from build123d import *

# Parameters (mm, degrees)
MOUNT_SKETCH_W       = 18
MOUNT_SKETCH_H       = 7.25
PIN_HOLE_SKETCH_W    = 3
PIN_HOLE_SKETCH_H    = 9.25
PIN_HOLES_X2_COUNT   = 2
SCREW_HOLE_SKETCH_W  = 1.65
SCREW_HOLE_SKETCH_H  = 9.25
SCREW_HOLES_X8_COUNT = 8


with BuildPart() as part:
    # Mount Sketch → Mount (revolve)
    with BuildSketch(Plane.XY, mode=Mode.PRIVATE) as mount_sk:
        with Locations((-48, 95.625)):
            Rectangle(MOUNT_SKETCH_W, MOUNT_SKETCH_H)
    revolve(mount_sk.sketch.rotate(Axis((-108, 0, 0), (1, 0, 0)), 90), axis=Axis((-108, 0, 0), (1, 0, 0)))

    # Pin Hole Sketch → Pin Hole (revolve, cut)
    with BuildSketch(Plane.XY, mode=Mode.PRIVATE) as pin_hole_sk:
        with Locations((-46.5, 95.625)):
            Rectangle(PIN_HOLE_SKETCH_W, PIN_HOLE_SKETCH_H)
    pin_hole = revolve(pin_hole_sk.sketch.rotate(Axis((-48, 82, 0), (0, 1, 0)), 90), axis=Axis((-48, 82, 0), (0, 1, 0)), mode=Mode.SUBTRACT)

    # Pin Holes x2: Pin Hole ×2 about axis
    pin_holes_x2_axis = Axis((-38.1, 0, 0), (-1, 0, 0))
    for i in range(1, PIN_HOLES_X2_COUNT):
        add(pin_hole.rotate(pin_holes_x2_axis, i * 360 / PIN_HOLES_X2_COUNT), mode=Mode.SUBTRACT)

    # Screw Hole Sketch → Screw Hole (revolve, cut)
    with BuildSketch(Plane.XY, mode=Mode.PRIVATE) as screw_hole_sk:
        with Locations((-41.175, 95.625)):
            Rectangle(SCREW_HOLE_SKETCH_W, SCREW_HOLE_SKETCH_H)
    screw_hole = revolve(screw_hole_sk.sketch.rotate(Axis((-42, 82, 0), (0, 1, 0)), 90), axis=Axis((-42, 82, 0), (0, 1, 0)), mode=Mode.SUBTRACT)

    # Screw Holes x8: Screw Hole ×8 about axis
    screw_holes_x8_axis = Axis((-38.1, 0, 0), (-1, 0, 0))
    for i in range(1, SCREW_HOLES_X8_COUNT):
        add(screw_hole.rotate(screw_holes_x8_axis, i * 360 / SCREW_HOLES_X8_COUNT), mode=Mode.SUBTRACT)


solid = part.part
Here's how the part is built. I have some questions about the finished solid (model axes, mm). Coordinates: 2 decimals unless noted, no trailing zeros. Order: outer loops, then holes, each group sorted by start corner. A loop starts at its lowest first (then second) coordinate and runs counter-clockwise, first axis right, second up.
Item 1: If we section it at B-B on z = 19.5: List the corners of the cut face in (x, y) for me, plus the area to 3 significant figures.
Result sheet:
outline: (-57, -97.32) - (-39, -97.32) - (-39, -89.91) - (-57, -89.91) - close; (-57, 89.91) - (-39, 89.91) - (-39, 97.32) - (-57, 97.32) - close
area: 267 mm2
Item 2: For P1, Ø5, axis at x = -44, y = 44, coming from the -Z side; P2, Ø2, axis at x = -43.5, z = 60.5, coming from the +Y side; P3, Ø5, axis at x = -52.5, y = 15.5, coming from the +Z side; P4, Ø3.5, axis at x = -48, z = 0, coming from the +Y side, each with a flat end and sliding along its axis, tell me the tip position at first contact or that it passes through.
Result sheet:
P1: stops at z = -90.16
P2: stops at y = 79.44
P3: stops at z = 98.39
P4: passes through
Item 3: If we section it at A-A on y = 29: List the corners of the cut face in (x, z) for me, plus the area to 3 significant figures.
Result sheet:
outline: (-57, -94.92) - (-39, -94.92) - (-39, -87.31) - (-57, -87.31) - close; (-57, 87.31) - (-39, 87.31) - (-39, 94.92) - (-57, 94.92) - close
area: 274 mm2
Item 4: I need wall thicknesses on line 1 (X direction, y = 94, z = 0); line 2 (Y direction, x = -52.5, z = -40); line 3 (Z direction, x = -40, y = -64). Which ranges of each line are inside material? Lowest first, please.
Result sheet:
line 1: x = -57 to -51, -45 to -43.65, -40.35 to -39
line 2: y = -90.83 to -82.85, 82.85 to 90.83
line 3: z = -75.86 to -66.09, 66.09 to 75.86
Item 5: If we mould it in two halves opening along Y, with no side actions, what happens to faces 1 (the face through (-39, 29, -88)), 2 (the face through (-47.874, -29.812, 94.667)), 3 (the face through (-43.636, -67.8, 67.496))? For each: +Y half, -Y half, draft (parallel to the pull), parting line (faces both ways), or undercut.
Result sheet:
face 1: draft
face 2: parting line
face 3: undercut
